Design review of the part built by this model. Coordinates are the model's own, in mm. A direction names the side the tool comes from. Coordinates: 2 decimals unless noted, no trailing zeros. Order: outer loops, then holes, each group sorted by start corner. A loop starts at its lowest first (then second) coordinate and runs counter-clockwise, first axis right, second up. Notation, with made-up numbers: M 47.5,38.25 L 89.5,38.25 A11 ccw 89.5,50.25 Z; hole C 47,58.5 d2. An arc over 180 degrees is marked long. Use CSV: the item, a comma, the result in double quotes.
```python
from build123d import *

# Parameters (mm, degrees)
BOSS_EXTRUDE1_DEPTH         = 6.35
SKETCH2_W                   = 21.336
SKETCH2_H                   = 46.355
BOSS_EXTRUDE2_DEPTH         = 22.225
CUT_EXTRUDE1_DEPTH          = 99.476196362
CUT_EXTRUDE1_DEPTH_BACK     = 57.531
F_10_32_TAPPED_HOLE1_REACH  = 100.678
F_10_32_TAPPED_HOLE1_BORE_R = 2.0193
F_10_32_TAPPED_HOLE2_D      = 4.0386


with BuildPart() as part:
    # Sketch1 → Boss-Extrude1 (new body)
    with BuildSketch(Plane.XY):
        with BuildLine():
            Line((2.54, 0), (55.5625, 0))
            ThreePointArc((55.5625, 0), (80.9625, 25.4), (55.5625, 50.8))
            Line((55.5625, 50.8), (2.54, 50.8))
            ThreePointArc((2.54, 50.8), (0.743948776, 50.056051224), (0, 48.26))
            Line((0, 48.26), (0, 2.54))
            ThreePointArc((0, 2.54), (0.743948776, 0.743948776), (2.54, 0))
        make_face()
        with BuildLine():
            Line((66.724781353, 27.178), (70.280781353, 27.178))
            Line((70.280781353, 27.178), (70.280781353, 23.622))
            Line((70.280781353, 23.622), (66.724781353, 23.622))
            ThreePointArc((66.724781353, 23.622), (44.2595, 25.4), (66.724781353, 27.178))
        make_face(mode=Mode.SUBTRACT)
    extrude(amount=BOSS_EXTRUDE1_DEPTH)

    # Sketch2 → Boss-Extrude2 (add)
    with BuildSketch(Plane.XY.offset(6.35)):
        with Locations((12.2555, 25.4635)):
            Rectangle(SKETCH2_W, SKETCH2_H)
    extrude(amount=BOSS_EXTRUDE2_DEPTH)

    # Sketch3 → Cut-Extrude1 (cut, two sides: drawn at the far end of the back side and taken through both)
    with BuildSketch(Plane.ZY.offset(-1.5875).offset(-CUT_EXTRUDE1_DEPTH_BACK)):
        with BuildLine():
            Line((140.654563204, 8.636), (28.575, 8.636))
            ThreePointArc((28.575, 8.636), (11.7475, 25.4635), (28.575, 42.291))
            Line((28.575, 42.291), (140.654563204, 42.291))
            Line((140.654563204, 42.291), (364.813689613, 42.291))
            Line((364.813689613, 42.291), (364.813689613, 8.636))
            Line((364.813689613, 8.636), (140.654563204, 8.636))
        make_face()
    extrude(amount=CUT_EXTRUDE1_DEPTH + CUT_EXTRUDE1_DEPTH_BACK, mode=Mode.SUBTRACT)

    # #10-32 Tapped Hole1 bore → #10-32 Tapped Hole1 (cut, up to next)
    with BuildSketch(Plane(origin=(0, 48.641, 0), x_dir=(1, 0, 0), z_dir=(0, 1, 0)), mode=Mode.PRIVATE) as f_10_32_tapped_hole1_sk1:
        with Locations((12.2555, -17.4625)):
            Circle(F_10_32_TAPPED_HOLE1_BORE_R)
    f_10_32_tapped_hole1_tool1 = extrude(f_10_32_tapped_hole1_sk1.sketch, amount=-F_10_32_TAPPED_HOLE1_REACH, mode=Mode.PRIVATE) & part.part
    add(f_10_32_tapped_hole1_tool1.solids().sort_by_distance((12.2555, 48.641, 17.4625))[0], mode=Mode.SUBTRACT)

    # #10-32 Tapped Hole2 (through all)
    with Locations(Plane(origin=(0, 2.286, 0), x_dir=(-1, 0, 0), z_dir=(0, -1, 0))):
        with Locations((-12.2555, -17.4625)):
            Hole(F_10_32_TAPPED_HOLE2_D / 2)


solid = part.part
```
(1) Clearance check with flat-ended pins moving along their axes: P1, Ø1.5, axis at y = 10, z = 10.5, coming from the -X side; P2, Ø1.1, axis at x = 68, z = 4, coming from the -Y side; P3, Ø10, axis at y = 9.5, z = 4, coming from the +X side. State where each tip first meets the part, or that it passes through.
The answers:
P1,"stops at x = 1.59"
P2,"stops at y = 2.95"
P3,"stops at x = 78.5"
(2) For faces 4 (the face through (68, 27.178, 3)), 5 (the face through (22.923, 25, 10)), 6 (the face through (0.724, 0.764, 3.131)), list the 3-axis set-ups (+Z, -Z, +X, -X, +Y, -Y) from which the entire face can be reached by the end or side of a thin tool; tool diameter is ignored.
The answers:
face 4,"+Z, -Z"
face 5,"+Z, +X, +Y, -Y"
face 6,"+Z, -Z, -X, -Y"
(3) Add section A-A on x = 11.5. Give the number of separate pieces and of enclosed holes in the cut face, and give its area (3 significant figures).
The answers:
separate pieces,"3"
enclosed holes,"0"
area,"828 mm2"
(4) Add section C-C on y = 25.4. State the section outline as (x, z) points.
The answers:
outline,"M 0,0 L 44.26,0 L 44.26,6.35 L 22.92,6.35 L 22.92,11.75 L 1.59,11.75 L 1.59,6.35 L 0,6.35 Z; M 70.28,0 L 80.96,0 L 80.96,6.35 L 70.28,6.35 Z"
(5) Add section D-D on x = 47. State the section outline as (y, z) points, and give its area (3 significant figures).
The answers:
outline,"M 0,0 L 18.02,0 L 18.02,6.35 L 0,6.35 Z; M 32.78,0 L 50.8,0 L 50.8,6.35 L 32.78,6.35 Z"
area,"229 mm2"
(6) Add section B-B on z = 4.25. State the section outline as (x, y) points.
The answers:
outline,"M 0,2.54 A2.54 ccw 2.54,0 L 55.56,0 A25.4 ccw 55.56,50.8 L 2.54,50.8 A2.54 ccw 0,48.26 Z; hole M 66.72,23.62 L 70.28,23.62 L 70.28,27.18 L 66.72,27.18 A11.3 ccw long Z"
(7) The part is to be moulded in two halves that separate along X. For faces 1 (the face through (10, 2.286, 17)), 2 (the face through (1.588, 25, 10)), 3 (the face through (70.281, 25, 3)), say which applies: pulls with the +X half, pulls with the -X half, needs draft (parallel to the pull), parting line crosses it, or undercut.
The answers:
face 1,"needs draft"
face 2,"pulls with the -X half"
face 3,"undercut"
(8) Wall thickness on probe 1 along X at (y, z) = (25.4, 1.75); probe 2 along Z at (x, y) = (64, 41.5); probe 3 along X at (y, z) = (13, 10): over which ranges is each line inside the solid? List them lowest first.
The answers:
probe 1,"x = 0 to 44.26, 70.28 to 80.96"
probe 2,"z = 0 to 6.35"
probe 3,"x = 1.59 to 22.92"
